For this review, take the finished solid that the model builds, in its own axes (mm). Face numbers are marked on the shaded views. A direction names the side the tool comes from. Coordinates: 2 decimals unless noted, no trailing zeros. Loops run counter-clockwise (first coordinate to the right, second up) from the corner with the lowest first, then second, coordinate; pieces in that order, holes last. Notation, with made-up numbers: (41.25, 82.5) - (81.25, 82.5) arc R18 ccw to (81.25, 86.5) - close; hole circle Ø2 at (89.25, 79). An arc over 180 degrees is marked (long way). Answer as a JSON object with one key per item and string values. Group by question number.
Item 1: Tool access review of the marked faces 1 and 2: name each direction out of +Z, -Z, +X, -X, +Y, -Y from which nothing blocks a thin tool from reaching the whole face with its end or side.
Item 2: We need section A-A (x = 0). Give the boundary of the cut face in (y, z).
Item 3: We need section B-B (y = 21). Give the boundary of the cut face in (x, z), then the cut area to 3 significant figures.
Item 4: We need section D-D (z = -10). Give the boundary of the cut face in (x, y), then the cut area to 3 significant figures.
Item 5: Mouldability with a two-part tool opening along X and no side actions: class the marked faces 3, 4 and 5 as released by +X, released by -X, zero draft, split by the parting line, or undercut.
Item 6: Clearance check with flat-ended pins moving along their axes: pin 1 (4 mm diameter, centred on y = 12.5, z = 39, fed in from +X); pin 2 (1.5 mm diameter, centred on y = 7, z = 25.5, fed in from +X); pin 3 (3 mm diameter, centred on y = 43, z = 42.5, fed in from +X); pin 4 (2 mm diameter, centred on x = 11.5, z = 37, fed in from -Y). State where each tip first meets the part, or that it passes through.
Item 7: To check wall thickness, follow line 1 (Y direction, x = 0, z = 3); line 2 (Z direction, x = 22.5, y = 41); line 3 (Y direction, x = -7.5, z = 19.5). State the ranges of each line that lie inside material, in increasing order.
Item 8: We need section C-C (y = 3). Give the boundary of the cut face in (x, z), then the cut area to 3 significant figures.
from build123d import *

# Parameters (mm, degrees)
F1_DEPTH = 50
F3_DEPTH = 50.4
F4_R     = 10.712345
F5_DEPTH = 50
F6_DEPTH = 10


with BuildPart() as f1:
    # F0 (on Front) → F1 (new body)
    with BuildSketch(Plane.XZ):
        Polygon((-50.462149, 58.360573), (-50.462149, 22.817668), (-39.930917, 22.817668), align=None)
        Polygon((-39.930917, 22.817668), (-50.462149, 22.817668), (-50.462149, -22.817668), (50.462149, -22.817668), (50.462149, 22.817668), align=None)
    extrude(amount=-F1_DEPTH)

    # F2 (on Right) → F3 (join)
    with BuildSketch(Plane.YZ):
        Polygon((39.464, 22.817668), (50, 22.817668), (50, 58.360573), align=None)
    extrude(amount=-F3_DEPTH)

    # F4 (on face) → F5 (cut)
    with BuildSketch(Plane.XY.offset(22.817668)):
        with Locations((0, 22.833524)):
            Circle(F4_R)
    extrude(amount=-F5_DEPTH, mode=Mode.SUBTRACT)

    # F3_face (on face) → F6 (join)
    with BuildSketch(Plane(origin=(0, 46.488, 34.665303), x_dir=(0, 1, 0), z_dir=(1, 0, 0))):
        Polygon((-7.024, -11.847635), (3.512, -11.847635), (3.512, 23.69527), align=None)
    extrude(amount=F6_DEPTH)


solid = f1.part
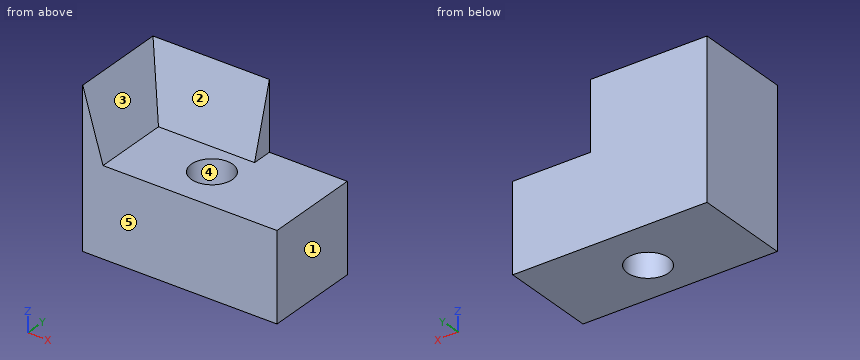
Check sheet entries:
{
 "1": {"face 1": "+Z, -Z, +X, +Y, -Y", "face 2": "+Z, +X, -Y"},
 "2": {"outline": "(0, -22.82) - (12.12, -22.82) - (12.12, 22.82) - (0, 22.82) - close; (33.55, -22.82) - (50, -22.82) - (50, 58.36) - (39.46, 22.82) - (33.55, 22.82) - close"},
 "3": {"outline": "(-50.46, -22.82) - (-10.55, -22.82) - (-10.55, 22.82) - (-39.93, 22.82) - (-50.46, 58.36) - close; (10.55, -22.82) - (50.46, -22.82) - (50.46, 22.82) - (10.55, 22.82) - close", "area": "3,830 mm2"},
 "4": {"outline": "(-50.46, 0) - (50.46, 0) - (50.46, 50) - (-50.46, 50) - close; hole circle Ø21.42 at (0, 22.83)", "area": "4,690 mm2"},
 "5": {"face 3": "released by +X", "face 4": "undercut", "face 5": "zero draft"},
 "6": {"pin 1": "stops at x = -44.13", "pin 2": "stops at x = -40.5", "pin 3": "stops at x = -45.32", "pin 4": "passes through"},
 "7": {"line 1": "y = 0 to 12.12, 33.55 to 50", "line 2": "z = -22.82 to 22.82", "line 3": "y = 0 to 15.18, 30.48 to 50"},
 "8": {"outline": "(-50.46, -22.82) - (50.46, -22.82) - (50.46, 22.82) - (-39.93, 22.82) - (-50.46, 58.36) - close", "area": "4,790 mm2"}
}
